For this review, take the finished solid that the model builds, in its own axes (mm). Give positions to 0.01 mm unless a question says otherwise; leave off trailing zeros. Order: outer loops, then holes, each group sorted by start corner. A loop starts at its lowest first (then second) coordinate and runs counter-clockwise, first axis right, second up. Notation, with made-up numbers: M 32,-5.75 L 76,-5.75 A15 ccw 76,0.25 Z; hole C -3,-8 d1. An arc over 180 degrees is marked long. Answer as CSV lines item,"result". Start each with the question number.
1. For line 1 along Z through (x, y) = (0, 1.5); line 2 along Z through (x, y) = (-2.5, 0.2), list the stretches that pass through material, from the lowest coordinate up.
2. We need section A-A, the plane z = 0. Give the boundary of the cut face in (x, y), and give its area (3 significant figures).
3. We need section C-C, the plane z = -34.5. Give the boundary of the cut face in (x, y).
4. We need section B-B, the plane x = 0. Give the boundary of the cut face in (y, z), and give its area (3 significant figures).
5. We need section D-D, the plane y = 0.85. Give the boundary of the cut face in (x, z), and give its area (3 significant figures).
6. Clearance check with flat-ended pins moving along their axes: P1, Ø1.3, axis at y = 0.5, z = 32, coming from the +X side; P2, Ø1, axis at x = 23.5, y = 1, coming from the +Z side. State where each tip first meets the part, or that it passes through.
from build123d import *

# Parameters (mm, degrees)
SKETCH1_W           = 31.75
SKETCH1_H           = 41.275
SKETCH1_W_2         = 41.275
SKETCH1_H_2         = 31.75
BOSS_EXTRUDE1_DEPTH = 2.54
SKETCH2_R           = 5.08
CUT_EXTRUDE1_DEPTH  = 2.54


with BuildPart() as part:
    # Sketch1 → Boss-Extrude1 (new body)
    with BuildSketch(Plane(origin=(0, 0, 0), x_dir=(1, 0, 0), z_dir=(0, 1, 0))):
        with Locations((-36.5125, 0)):
            Rectangle(SKETCH1_W, SKETCH1_H)
        Rectangle(SKETCH1_W_2, SKETCH1_H)
        with Locations((0, -36.5125)):
            Rectangle(SKETCH1_W_2, SKETCH1_H_2)
        with Locations((0, 36.5125)):
            Rectangle(SKETCH1_W_2, SKETCH1_H_2)
        with Locations((36.5125, 0)):
            Rectangle(SKETCH1_W, SKETCH1_H)
    extrude(amount=BOSS_EXTRUDE1_DEPTH)

    # Sketch2 → Cut-Extrude1 (cut)
    with BuildSketch(Plane(origin=(0, 2.54, 0), x_dir=(1, 0, 0), z_dir=(0, 1, 0))):
        with Locations((0, -36.5125)):
            Circle(SKETCH2_R)
        with Locations((-36.5125, 0)):
            Circle(SKETCH2_R)
        with Locations((0, 36.5125)):
            Circle(SKETCH2_R)
        with Locations((36.5125, 0)):
            Circle(SKETCH2_R)
    extrude(amount=-CUT_EXTRUDE1_DEPTH, mode=Mode.SUBTRACT)


solid = part.part
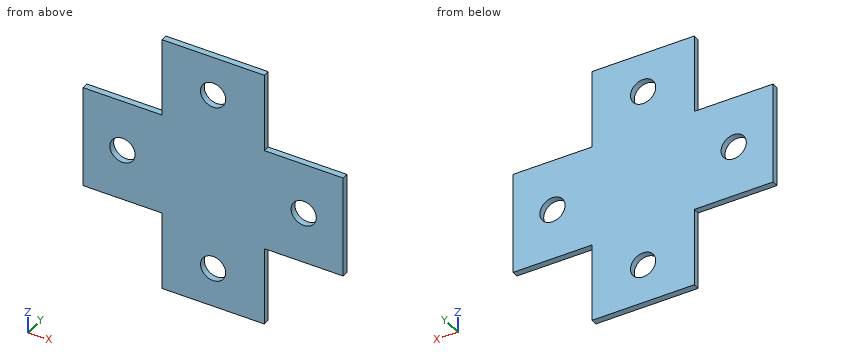
Result set:
1,line 1,"-52.39 to -41.59, -31.43 to 31.43, 41.59 to 52.39"
1,line 2,"-52.39 to -40.93, -32.09 to 32.09, 40.93 to 52.39"
2,outline,"M -52.39,0 L -41.59,0 L -41.59,2.54 L -52.39,2.54 Z; M -31.43,0 L 31.43,0 L 31.43,2.54 L -31.43,2.54 Z; M 41.59,0 L 52.39,0 L 52.39,2.54 L 41.59,2.54 Z"
2,area,"215 mm2"
3,outline,"M -20.64,0 L -4.66,0 L -4.66,2.54 L -20.64,2.54 Z; M 4.66,0 L 20.64,0 L 20.64,2.54 L 4.66,2.54 Z"
4,outline,"M 0,-52.39 L 2.54,-52.39 L 2.54,-41.59 L 0,-41.59 Z; M 0,-31.43 L 2.54,-31.43 L 2.54,31.43 L 0,31.43 Z; M 0,41.59 L 2.54,41.59 L 2.54,52.39 L 0,52.39 Z"
4,area,"215 mm2"
5,outline,"M -52.39,-20.64 L -20.64,-20.64 L -20.64,-52.39 L 20.64,-52.39 L 20.64,-20.64 L 52.39,-20.64 L 52.39,20.64 L 20.64,20.64 L 20.64,52.39 L -20.64,52.39 L -20.64,20.64 L -52.39,20.64 Z; hole C -36.51,0 d10.16; hole C 0,-36.51 d10.16; hole C 0,36.51 d10.16; hole C 36.51,0 d10.16"
5,area,"6,620 mm2"
6,P1,"x = 20.64"
6,P2,"z = 20.64"
